Autodesk Inventor part; units mm, degrees
ref_plane "YZ Plane" through (0, 0, 0) normal (1, 0, 0) x (0, 1, 0)
ref_plane "XZ Plane" through (0, 0, 0) normal (0, 1, 0) x (-1, 0, 0)
ref_plane "XY Plane" through (0, 0, 0) normal (0, 0, 1) x (1, 0, 0)
sketch "Sketch1" plane through (0, 0, 0) normal (0, 1, 0) x (-1, 0, 0)
  line L0 (0, 0) -> (0, -8.382)
  line L1 (0, -8.382) -> (0, -9.398)
  line L2 (0, -9.398) -> (0, -13.208)
  line L3 (0, -8.382) -> (2.54, -8.382)
  line L4 (2.54, -8.382) -> (0, 0)
  line L5 (0, -9.398) -> (1.651, -9.398)
  line L6 (1.651, -9.398) -> (1.651, -8.382)
  line L7 (0, -13.208) -> (1.905, -13.208)
  line L8 (1.905, -13.208) -> (1.905, -9.398)
  line L9 (1.905, -9.398) -> (1.651, -9.398)
  line L10 (0, 0) -> (0, -1.016)
  line L11 (1.651, -8.382) -> (1.397, -8.382)
  line L12 (0, -1.016) -> (1.397, -8.382)
  line L13 (1.397, -8.382) -> (1.397, -13.208)
  dimension "d0" = 8.382
  dimension "d1" = 1.016
  dimension "d2" = 3.81
  dimension "d3" = 2.54
  dimension "d4" = 1.651
  dimension "d5" = 1.905
  dimension "d6" = 1.016
  dimension "d7" = 0.254
revolve "Revolution1" add sketch "Sketch1" angle 360 about axis through (0, 0, 0) along (0, 0, -1) contours L4 L3 L12 L0 | L3 L6 L5 L13 | L5 L9 L8 L7 L13
properties part number "Pencil Tip"
Work out the finished part from the listing and answer in its coordinate system (mm). A direction names the side the tool comes from. Round coordinates to 2 decimals unless told otherwise and drop trailing zeros. Write each loop counter-clockwise with the first axis right and the second up, starting at its lowest first coordinate (ties: lowest second). Pieces come first, ordered by that corner, then holes. Notation, with made-up numbers: (0, -9.75) -> (49, -9.75) arc R27 ccw to (49, 12.25) -> close; hole circle Ø8 at (67, 45). An arc over 180 degrees is marked (long way). Write each question's results on one line, items separated by ' | '.
Q1. Section B-B, the plane z = -5 is taken. Write down the section's boundary in (x, y), then the cut area to 3 significant figures.
Data:
outline: circle Ø3.03 at (0, 0); hole circle Ø1.51 at (0, 0) | area: 5.42 mm^2
Q2. Section A-A, the plane z = -7 is taken. Write down the section's boundary in (x, y), then the cut area to 3 significant figures.
Data:
outline: circle Ø4.24 at (0, 0); hole circle Ø2.27 at (0, 0) | area: 10.1 mm^2
Q3. Determine the mould class of faces 3 (the cylindrical face through (1.11, -0.85, -10.83)), 4 (the flat face through (0, -2, -8.382)), 5 (the conical face through (1.022, -0.784, -4.25)) for opening direction Z: released by +Z, released by -Z, zero draft, split by the parting line, or undercut.
Data:
face 3: zero draft | face 4: undercut | face 5: released by +Z
Q4. Straight lines are drawn through the part: line 1 along Y through (x, z) = (0, -9.45) (3 decimals); line 2 along X through (y, z) = (-0.05, -9.75); line 3 along Y through (x, z) = (0.1, -6). For each, find the intervals that lie inside material, in ascending order. Write a range as [from, to].
Data:
line 1: [-1.905, -1.397], [1.397, 1.905] | line 2: [-1.9, -1.4], [1.4, 1.9] | line 3: [-1.82, -0.94], [0.94, 1.82]
Q5. Which of the six approach directions +Z, -Z, +X, -X, +Y, -Y give full straight-line access (tool end or side, diameter ignored) to faces 1 (the cylindrical face through (-1.525, 0.632, -8.883)), 2 (the cylindrical face through (0.41, 1.86, -11.28))?
Data:
face 1: none | face 2: -Z
